Geometry check sheet. Reference: the model listing, model coordinates, mm. Face numbers are marked on the shaded views. A direction names the side the tool comes from. Round coordinates to 2 decimals unless told otherwise and drop trailing zeros. Order: outer loops, then holes, each group sorted by start corner. A loop starts at its lowest first (then second) coordinate and runs counter-clockwise, first axis right, second up.
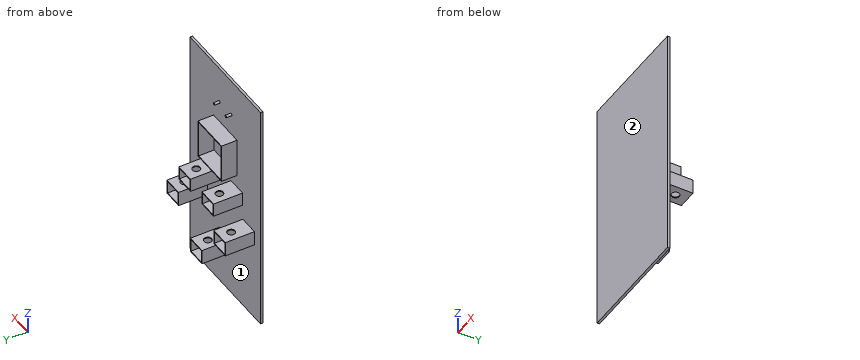
```python
from build123d import *

# Parameters (mm, degrees)
SKETCH1_W           = 304.8
SKETCH1_H           = 609.6
BOSS_EXTRUDE1_DEPTH = 6.35
SKETCH2_W           = 50
SKETCH2_H           = 38
BOSS_EXTRUDE2_DEPTH = 75
SKETCH4_W           = 50.000000076
SKETCH4_H           = 37.999999946
BOSS_EXTRUDE3_DEPTH = 75
SKETCH5_W           = 50
SKETCH5_H           = 35
BOSS_EXTRUDE4_DEPTH = 75
SHELL11_T           = -2.54
SKETCH3_R           = 10
CUT_EXTRUDE2_DEPTH  = 75
SKETCH6_R           = 10
CUT_EXTRUDE3_DEPTH  = 75
SKETCH7_R           = 10
CUT_EXTRUDE4_DEPTH  = 75
SKETCH8_W           = 101.6
SKETCH8_H           = 101.6
BOSS_EXTRUDE5_DEPTH = 40
SHELL12_START       = 6.35
SHELL12_OUTLINE_W   = 96.52
SHELL12_OUTLINE_H   = 96.52
SHELL12_DEPTH       = 40
SKETCH9_R           = 3.16
BOSS_EXTRUDE6_DEPTH = 13.8176


# Read off the part's stored shape, not the designer's step: Shell12
with BuildPart() as part:
    # Sketch1 → Boss-Extrude1 (new body)
    with BuildSketch(Plane(origin=(0, 0, 0), x_dir=(1, 0, 0), z_dir=(0, 1, 0))):
        Rectangle(SKETCH1_W, SKETCH1_H)
    extrude(amount=BOSS_EXTRUDE1_DEPTH)

    # Sketch2 → Boss-Extrude2 (add)
    with BuildSketch(Plane(origin=(0, 6.35, 0), x_dir=(1, 0, 0), z_dir=(0, 1, 0))):
        with Locations((0, 171.4)):
            Rectangle(SKETCH2_W, SKETCH2_H)
    extrude(amount=BOSS_EXTRUDE2_DEPTH)

    # Sketch4 → Boss-Extrude3 (add)
    with BuildSketch(Plane(origin=(0, 6.35, 0), x_dir=(1, 0, 0), z_dir=(0, 1, 0))):
        with Locations((-101.200000038, 76.2)):
            Rectangle(SKETCH4_W, SKETCH4_H)
    boss_extrude3 = extrude(amount=BOSS_EXTRUDE3_DEPTH)

    # Sketch5 → Boss-Extrude4 (add)
    with BuildSketch(Plane(origin=(0, 6.35, 0), x_dir=(1, 0, 0), z_dir=(0, 1, 0))):
        with Locations((-50, 0)):
            Rectangle(SKETCH5_W, SKETCH5_H)
    boss_extrude4 = extrude(amount=BOSS_EXTRUDE4_DEPTH)

    # Mirror1: Boss-Extrude3, Boss-Extrude4 across plane
    add(boss_extrude3.mirror(Plane(origin=(0, 0, 0), x_dir=(0, 0, 1), z_dir=(1, 0, 0))))
    add(boss_extrude4.mirror(Plane(origin=(0, 0, 0), x_dir=(0, 0, 1), z_dir=(1, 0, 0))))

    # Shell11
    shell11_openings = [part.faces().sort_by_distance(p)[0] for p in [
        (0, 81.35, -171.4),
        (-101.200000038, 81.35, -76.2),
        (-50, 81.35, 0),
        (101.200000038, 81.35, -76.2),
        (50, 81.35, 0),
    ]]
    offset(amount=SHELL11_T, openings=shell11_openings, kind=Kind.INTERSECTION)

    # Sketch3 → Cut-Extrude2 (cut)
    with BuildSketch(Plane.XY.offset(-152.4)):
        with Locations((0, 51.35)):
            Circle(SKETCH3_R)
    extrude(amount=-CUT_EXTRUDE2_DEPTH, mode=Mode.SUBTRACT)

    # Sketch6 → Cut-Extrude3 (cut)
    with BuildSketch(Plane.XY.offset(-57.200000027)):
        with Locations((-101.2, 51.35)):
            Circle(SKETCH6_R)
    cut_extrude3 = extrude(amount=-CUT_EXTRUDE3_DEPTH, mode=Mode.SUBTRACT)

    # Sketch7 → Cut-Extrude4 (cut)
    with BuildSketch(Plane.XY.offset(17.5)):
        with Locations((-50, 51.35)):
            Circle(SKETCH7_R)
    cut_extrude4 = extrude(amount=-CUT_EXTRUDE4_DEPTH, mode=Mode.SUBTRACT)

    # Mirror2: Cut-Extrude3, Cut-Extrude4 across plane
    add(cut_extrude3.mirror(Plane(origin=(0, 0, 0), x_dir=(0, 0, 1), z_dir=(1, 0, 0))), mode=Mode.SUBTRACT)
    add(cut_extrude4.mirror(Plane(origin=(0, 0, 0), x_dir=(0, 0, 1), z_dir=(1, 0, 0))), mode=Mode.SUBTRACT)

    # Sketch8 → Boss-Extrude5 (add)
    with BuildSketch(Plane(origin=(0, 6.35, 0), x_dir=(1, 0, 0), z_dir=(0, 1, 0))):
        with Locations((0, -101.6)):
            Rectangle(SKETCH8_W, SKETCH8_H)
    extrude(amount=BOSS_EXTRUDE5_DEPTH)

    # Shell12 outline → Shell12 (cut)
    with BuildSketch(Plane(origin=(0, 0, 0), x_dir=(1, 0, 0), z_dir=(0, 1, 0)).offset(SHELL12_START)):
        with Locations((0, -101.6)):
            Rectangle(SHELL12_OUTLINE_W, SHELL12_OUTLINE_H)
    extrude(amount=SHELL12_DEPTH, mode=Mode.SUBTRACT)

    # Sketch9 → Boss-Extrude6 (add)
    with BuildSketch(Plane(origin=(0, 6.35, 0), x_dir=(1, 0, 0), z_dir=(0, 1, 0))):
        with Locations(Location((-25.4, -208.456082319, 0), (0, 0, 90))):
            Circle(SKETCH9_R)
    boss_extrude6 = extrude(amount=BOSS_EXTRUDE6_DEPTH)

    # Mirror3: Boss-Extrude6 across plane
    add(boss_extrude6.mirror(Plane(origin=(0, 0, 0), x_dir=(0, 0, 1), z_dir=(1, 0, 0))))


solid = part.part
```
(1) Material ranges on line 1 (Y direction, x = -50, z = -15); line 2 (Z direction, x = -15.5, y = 29.5); line 3 (X direction, y = 51, z = 15), recorded low to high.
Returned:
line 1: y = 0 to 2.54, 3.81 to 41.35, 61.35 to 81.35
line 2: z = -190.4 to -187.86, -154.94 to -152.4, 50.8 to 53.34, 149.86 to 152.4
line 3: x = -75 to -59.99, -40.01 to -25, 25 to 40.01, 59.99 to 75
(2) Sectioned sample at D-D, the plane y = 73.5. Give the number of separate pieces and of enclosed holes in the cut face, and give its area (3 significant figures).
Returned:
separate pieces: 5
enclosed holes: 5
area: 2,080 mm2
(3) Depth check by flat-ended pin: P1, Ø16.5, axis at y = 43, z = -83.5, coming from the +X side; P2, Ø18, axis at x = 0, y = 51.35, coming from the +Z side; P3, Ø22.5, axis at x = 48.5, y = 60, coming from the -Z side. Enter the tip coordinate at first touch or a pass-through.
Returned:
P1: stops at x = 126.2
P2: stops at z = 152.4
P3: stops at z = -17.5
(4) Sectioned sample at C-C, the plane z = 261.5. Record the cut outline in (x, y).
Returned:
outline: (-152.4, 0) - (152.4, 0) - (152.4, 6.35) - (-152.4, 6.35) - close; hole (-149.86, 2.54) - (149.86, 2.54) - (149.86, 3.81) - (-149.86, 3.81) - close
(5) Set-up check for the marked faces 1 and 2: record each of +Z, -Z, +X, -X, +Y, -Y from which the full face is reachable in a straight line by a thin tool's end or side.
Returned:
face 1: +Y
face 2: +Z, -Z, +X, -X, -Y
(6) Sectioned sample at B-B, the plane z = -8.5. Record the cut outline in (x, y).
Returned:
outline: (-152.4, 0) - (152.4, 0) - (152.4, 6.35) - (75, 6.35) - (75, 81.35) - (72.46, 81.35) - (72.46, 3.81) - (149.86, 3.81) - (149.86, 2.54) - (-149.86, 2.54) - (-149.86, 3.81) - (-72.46, 3.81) - (-72.46, 81.35) - (-75, 81.35) - (-75, 6.35) - (-152.4, 6.35) - close; (-27.54, 3.81) - (27.54, 3.81) - (27.54, 81.35) - (25, 81.35) - (25, 6.35) - (-25, 6.35) - (-25, 81.35) - (-27.54, 81.35) - close
(7) Sectioned sample at A-A, the plane x = -101.2. Record the cut outline in (y, z).
Returned:
outline: (0, -304.8) - (6.35, -304.8) - (6.35, -95.2) - (41.35, -95.2) - (41.35, -92.66) - (3.81, -92.66) - (3.81, -302.26) - (2.54, -302.26) - (2.54, 302.26) - (3.81, 302.26) - (3.81, -59.74) - (41.35, -59.74) - (41.35, -57.2) - (6.35, -57.2) - (6.35, 304.8) - (0, 304.8) - close; (61.35, -95.2) - (81.35, -95.2) - (81.35, -92.66) - (61.35, -92.66) - close; (61.35, -59.74) - (81.35, -59.74) - (81.35, -57.2) - (61.35, -57.2) - close
